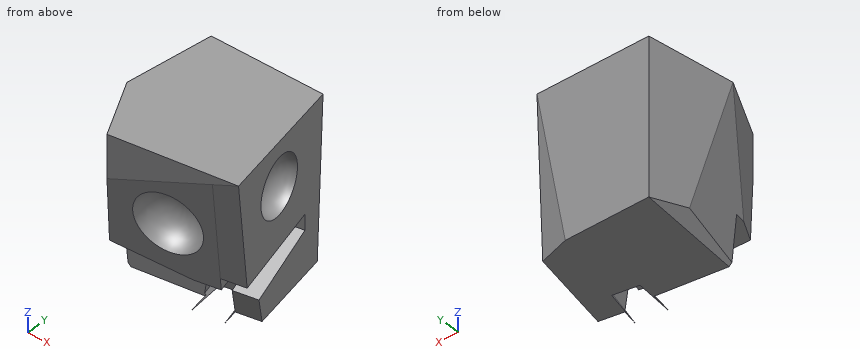
from build123d import *

# Parameters (mm, degrees)
F1_DEPTH  = 100
F6_DEPTH  = 25
F7_DEPTH  = 15
F9_DEPTH  = 25
F3_R      = 17.8601151659
F10_DEPTH = 13
F11_R     = 12.99999
F13_DEPTH = 25
F14_DEPTH = 90
F12_R     = 19.8108840593
F15_DEPTH = 17
F16_R     = 16.99999
F18_DEPTH = 25


# Not quite as in the source:
# - a fillet or chamfer is up to 0.001 mm smaller than in the source, because OpenCascade refuses the exact size


with BuildPart() as f1:
    # F0 (on Top) → F1 (new body)
    with BuildSketch(Plane.XY):
        Polygon((-47.5200526416, -19.4592215121), (-27.9358569533, -56.1545789242), (46.7044450343, -43.9518280327), (29.7740362585, 36.9222164154), (-40.8926419914, 34.7126610577), align=None)
    extrude(amount=F1_DEPTH)

    # F5 (on 3pt) → F6 (cut)
    with BuildSketch(Plane(origin=(9.6412332648, 36.848921293, -1.9307798529), x_dir=(0.9675193136, -0.2524507981, 0.0132277119), z_dir=(-0.2527971081, -0.9661938968, 0.0506258432))):
        Polygon((22.0081010682, 1.6419123086), (20.808683311, 101.7949787998), (2.3196212658, 1.9027031079), align=None)
    extrude(amount=-F6_DEPTH, mode=Mode.SUBTRACT)

    # F3 (on face) → F7 (cut)
    with BuildSketch(Plane(origin=(35.9288773181, 7.5214561607, 0), x_dir=(-0.2049012214, 0.9787826569, 0), z_dir=(0.9787826569, 0.2049012214, 0))):
        Polygon((-44.1726371646, 30.7864621282), (-52.589084849, 100), (-52.589084849, 0), (-29.6385996044, 0), (-32.5648710132, 15.3381312266), (12.4055901776, 27.6119541377), (12.4055901776, 37.6664411777), align=None)
    extrude(amount=-F7_DEPTH, mode=Mode.SUBTRACT)

    # F8 (on face) → F9 (cut)
    with BuildSketch(Plane(origin=(8.1632362237, -38.9945652191, -4.8445740248), x_dir=(0.979095124, 0.2018510885, 0.0250774059), z_dir=(0.2034028962, -0.9716253806, -0.1207119775))):
        Polygon((39.3641106636, 104.6558680882), (-79.5409610954, 107.6664552623), (-81.3024698416, 37.9594929491), (22.60753629, 35.3336665102), (24.2297143871, 99.5269938077), align=None)
        Polygon((22.60753629, 35.3336665102), (-81.3024698416, 37.9594929491), (-82.4683913698, -8.1787100022), (37.6027492107, -11.21293151), (37.6027492107, 34.9547345092), align=None)
    extrude(amount=F9_DEPTH, mode=Mode.SUBTRACT)

    # F3 (on face) → F10 (cut)
    with BuildSketch(Plane(origin=(35.9288773181, 7.5214561607, 0), x_dir=(-0.2049012214, 0.9787826569, 0), z_dir=(0.9787826569, 0.2049012214, 0))):
        with Locations((-12.8240771592, 72.3933577538)):
            Circle(F3_R)
    extrude(amount=-F10_DEPTH, mode=Mode.SUBTRACT)

    # F11 (radius 13 in the source; OpenCascade refuses exactly that, so slightly less here)
    f11_edges = [f1.edges().sort_by_distance(p)[0] for p in [
        (29.491931, -25.175415, 72.393358),
    ]]
    fillet(f11_edges, radius=F11_R)

    # F12 (on face) → F13 (cut)
    with BuildSketch(Plane(origin=(8.1632362237, -38.9945652191, -4.8445740248), x_dir=(0.979095124, 0.2018510885, 0.0250774059), z_dir=(0.2034028962, -0.9716253806, -0.1207119775))):
        Polygon((21.8240755779, 4.3303198355), (22.4123828022, 27.6109930646), (6.6332079808, 28.009735938), (2.6960770767, 4.8136881468), align=None)
        Polygon((18.9769355737, -4.4831562801), (21.8240755779, 4.3303198355), (2.6960770767, 4.8136881468), (9.4391942611, -4.4458445128), align=None)
    extrude(amount=-F13_DEPTH, mode=Mode.SUBTRACT)

    # F12 (on face) → F14 (cut)
    with BuildSketch(Plane(origin=(8.1632362237, -38.9945652191, -4.8445740248), x_dir=(0.979095124, 0.2018510885, 0.0250774059), z_dir=(0.2034028962, -0.9716253806, -0.1207119775))):
        Polygon((-50.4545168754, 2.399114297), (-41.2831704405, 5.9250524436), (-47.9467762851, 101.636191148), align=None)
        Polygon((-33.0309979628, -4.2797005717), (-41.2831704405, 5.9250524436), (-50.4545168754, 2.399114297), align=None)
    extrude(amount=-F14_DEPTH, mode=Mode.SUBTRACT)

    # F12 (on face) → F15 (cut)
    with BuildSketch(Plane(origin=(8.1632362237, -38.9945652191, -4.8445740248), x_dir=(0.979095124, 0.2018510885, 0.0250774059), z_dir=(0.2034028962, -0.9716253806, -0.1207119775))):
        with Locations((-4.2161699384, 61.7149807513)):
            Circle(F12_R)
    extrude(amount=-F15_DEPTH, mode=Mode.SUBTRACT)

    # F16 (radius 17 in the source; OpenCascade refuses exactly that, so slightly less here)
    f16_edges = [f1.edges().sort_by_distance(p)[0] for p in [
        (-18.819384, -34.935619, 57.849136),
    ]]
    fillet(f16_edges, radius=F16_R)

    # F17 (on face) → F18 (cut)
    with BuildSketch(Plane(origin=(8.2143401196, -50.2444762342, 0), x_dir=(0.9868979975, 0.1613454139, 0), z_dir=(0.1613454139, -0.9868979975, 0))):
        Polygon((7.8329915962, 23.1178128028), (-44.1760422775, 30.926933164), (-42.148109545, 7.0275762015), (-39.5882407468, 0), (4.361868039, 0), align=None)
    extrude(amount=-F18_DEPTH, mode=Mode.SUBTRACT)


solid = f1.part
Can you work these out from the model? Positions are in its coordinate system, mm. Give positions to 0.01 mm unless a question says otherwise; leave off trailing zeros. Order: outer loops, then holes, each group sorted by start corner. A loop starts at its lowest first (then second) coordinate and runs counter-clockwise, first axis right, second up. Notation, with made-up numbers: M -15,45 L -1,45 A19 ccw -1,49 Z; hole C 22.25,-0.5 d10. An arc over 180 degrees is marked long. Use one line per item in the form item = value. Start each with the question number.
Item 1: If I drill on line 1 along Z through (x, y) = (38, -18); line 2 along X through (y, z) = (20.5, 39.5); line 3 along Y through (x, z) = (0.5, 92), over which ranges is the centre line in solid material (lowest first)?
Item 2: If we section it at A-A (z = 13): Write out the boundary of the cut face in (x, y).
Item 3: If we section it at B-B (y = 26): Write out the boundary of the cut face in (x, z).
Item 4: Will these pins go through, and if not, where does the flat tip stop? pin 1 Ø12 at (y, z) = (24.5, 33) entering from -X; pin 2 Ø2 at (y, z) = (1.5, 52.5) entering from +X; pin 3 Ø8 at (x, y) = (-31, -37) entering from -Z.
Outcome:
q1.line_1 = 0 to 17.29, 33.07 to 60.29, 84.5 to 100
q1.line_2 = -42.63 to 33.21
q1.line_3 = -51.51 to 36.01
q2.outline = M -44.32,6.71 L -36.63,-32.24 L 9.45,-24.71 L 7.38,-15.64 L 24.69,-12.02 L 27.83,-26.99 L 42.51,-23.92 L 30.78,32.1 L 14.21,36.44 L -40.89,34.71 Z
q3.outline = M -41.96,2.34 L -39.98,0 L 32.06,0 L 32.06,100 L -41.96,100 Z
q4.pin_1 = -42.88
q4.pin_2 = 37.4
q4.pin_3 = 29.18
